Drawing for the job (mm, zero at the part's lowest x, y, z). Coordinates: 2 decimals unless noted, no trailing zeros. Loops run counter-clockwise (first coordinate to the right, second up) from the corner with the lowest first, then second, coordinate; pieces in that order, holes last. Notation, with made-up numbers: (77, 87) - (127, 87) arc R24 cw to (127, 104) - close; hole circle Ø6 at (21, 35.25). An arc over 180 degrees is marked (long way). One line per item, written item: value.
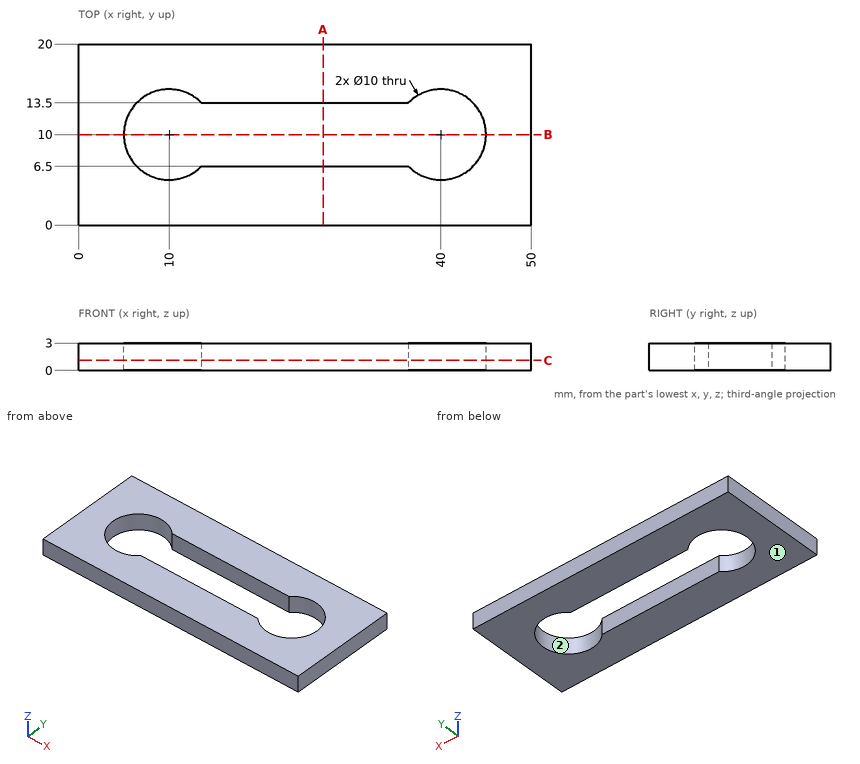
Item 1: Pull direction Y, two halves, no side cores. Call the marked faces 1 and 2: released by +Y, released by -Y, zero draft, split by the parting line, or undercut.
Check result:
face 1: zero draft
face 2: undercut
Item 2: Cut at B-B, the plane y = 10. Write the cut outline in (x, z).
Check result:
outline: (0, 0) - (5, 0) - (5, 3) - (0, 3) - close; (45, 0) - (50, 0) - (50, 3) - (45, 3) - close
Item 3: Cut at A-A, the plane x = 27. Write the cut outline in (y, z), then the cut area to 3 significant figures.
Check result:
outline: (0, 0) - (6.5, 0) - (6.5, 3) - (0, 3) - close; (13.5, 0) - (20, 0) - (20, 3) - (13.5, 3) - close
area: 39.0 mm^2
Item 4: Cut at C-C, the plane z = 1.1. Write the cut outline in (x, y), then the cut area to 3 significant figures.
Check result:
outline: (0, 0) - (50, 0) - (50, 20) - (0, 20) - close; hole (13.57, 6.5) - (36.43, 6.5) arc R5 ccw (long way) to (36.43, 13.5) - (13.57, 13.5) arc R5 ccw (long way) to start
area: 697 mm^2
Item 5: Probe probe 1 along Y at (x, z) = (18, 0.4); probe 2 along X at (y, z) = (13.75, 2.85); probe 3 along Y at (x, z) = (40, 1.9). List the from-to ranges inside material, lowest first. Write a range as from..to.
Check result:
probe 1: y = 0..6.5, 13.5..20
probe 2: x = 0..6.69, 13.31..36.69, 43.31..50
probe 3: y = 0..5, 15..20
